For this review, take the finished solid that the model builds, in its own axes (mm). A direction names the side the tool comes from. Round coordinates to 2 decimals unless told otherwise and drop trailing zeros. Write each loop counter-clockwise with the first axis right and the second up, starting at its lowest first coordinate (ties: lowest second). Pieces come first, ordered by that corner, then holes. Notation, with made-up numbers: (3, 0.5) - (55, 0.5) arc R6 ccw to (55, 4.5) - close; hole circle Ø10 at (51, -10.5). An arc over 180 degrees is marked (long way). One line per item, written item: value. Start each with the question number.
Q1. Tool access review of faces 1 (the face through (-0.847, 1.288, 15.297)), 2 (the face through (-3.141, 1.288, -14.995)), 3 (the face through (13, 1, -8.382)), 4 (the face through (-14.556, 1.288, -4.777)): name each direction out of +Z, -Z, +X, -X, +Y, -Y from which nothing blocks a thin tool from reaching the whole face with its end or side.
Q2. Clearance check with flat-ended pins moving along their axes: pin 1 Ø8 at (x, y) = (-2, 24) entering from -Z; pin 2 Ø0.8 at (y, z) = (1, -12.5) entering from -X; pin 3 Ø2 at (y, z) = (1.5, -13.5) entering from +X; pin 4 Ø8 at (x, y) = (-10, 14.5) entering from -Z. State where each tip first meets the part, or that it passes through.
Q3. Add section B-B on z = -9.5. Write out the cut boundary in (x, y).
Q4. Mouldability with a two-part tool opening along Z and no side actions: class faces 5 (the face through (14.601, 1.288, -4.765)), 6 (the face through (0, 0, 0)), 7 (the face through (6.91, 1.29, 13.67)) as +Z half, -Z half, draft (parallel to the pull), parting line (faces both ways), or undercut.
Q5. Add section A-A on y = 32.5. Write out the cut boundary in (x, z).
Q6. For probe 1 along Y at (x, z) = (11, 11); probe 2 along Z at (x, y) = (-2.5, 32); probe 3 along X at (y, z) = (11, 0.5), list the stretches that pass through material, from the lowest coordinate up.
Q7. Add section C-C on x = 6. Write out the cut boundary in (y, z).
```python
from build123d import *

# Parameters (mm, degrees)
SKETCH1_R           = 13.97
BOSS_EXTRUDE1_DEPTH = 2.54
BOSS_EXTRUDE2_DEPTH = 2.54
CIRPATTERN1_COUNT   = 24
SKETCH3_R           = 3.2385
BOSS_EXTRUDE3_DEPTH = 31.75


with BuildPart() as part:
    # Sketch1 → Boss-Extrude1 (new body)
    with BuildSketch(Plane(origin=(0, 0, 0), x_dir=(1, 0, 0), z_dir=(0, 1, 0))):
        with Locations(Location((0, 0, 0), (0, 0, 270))):
            Circle(SKETCH1_R)
    extrude(amount=BOSS_EXTRUDE1_DEPTH)

    # Sketch2 → Boss-Extrude2 (add)
    with BuildSketch(Plane(origin=(0, 2.54, 0), x_dir=(1, 0, 0), z_dir=(0, 1, 0))):
        Polygon((0, -16.764), (3.64730005, -10.446691002), (-3.581879589, -10.560002566), align=None)
    boss_extrude2 = extrude(amount=-BOSS_EXTRUDE2_DEPTH)

    # CirPattern1: Boss-Extrude2 ×24 about axis
    cirpattern1_axis = Axis((0, 0, 0), (0, 1, 0))
    for i in range(1, CIRPATTERN1_COUNT):
        add(boss_extrude2.rotate(cirpattern1_axis, i * 360 / CIRPATTERN1_COUNT))

    # Sketch3 → Boss-Extrude3 (add)
    with BuildSketch(Plane(origin=(0, 2.54, 0), x_dir=(1, 0, 0), z_dir=(0, 1, 0))):
        with Locations(Location((0, 0, 0), (0, 0, 270))):
            Circle(SKETCH3_R)
    extrude(amount=BOSS_EXTRUDE3_DEPTH)


solid = part.part
```
Result set:
1. face 1: +Z, +Y, -Y
1. face 2: -Z, +Y, -Y
1. face 3: +X, +Y, -Y
1. face 4: -X, +Y, -Y
2. pin 1: stops at z = -3.24
2. pin 2: stops at x = -8.38
2. pin 3: stops at x = 8.38
2. pin 4: passes through
3. outline: (-11.22, 0) - (11.22, 0) - (11.22, 2.54) - (-11.22, 2.54) - close
4. face 5: undercut
4. face 6: draft
4. face 7: +Z half
5. outline: circle Ø6.48 at (0, 0)
6. probe 1: y = 0 to 2.54
6. probe 2: z = -2.06 to 2.06
6. probe 3: x = -3.2 to 3.2
7. outline: (0, -13.14) - (2.54, -13.14) - (2.54, 13.14) - (0, 13.14) - close
